Check sheet for the modelled part. Datum: model origin and axes. Units: mm. Round coordinates to 2 decimals unless told otherwise and drop trailing zeros. Order: outer loops, then holes, each group sorted by start corner. A loop starts at its lowest first (then second) coordinate and runs counter-clockwise, first axis right, second up.
Q1. Cross-section at B-B on y = 2. Give the number of separate pieces and of enclosed holes in the cut face, then the cut area to 3 significant figures.
Q2. Scan lines: probe 1 along Z at (x, y) = (5, 3.5); probe 2 along Y at (x, z) = (10.5, 1.95); probe 3 along Y at (x, z) = (7.25, 2.05). Record each from-to range of solid material in increasing order.
Q3. Cross-section at A-A on x = 12.25. Record the cut outline in (y, z).
Q4. Depth check by flat-ended pin: P1, Ø1.2, axis at x = 2.5, z = 1, coming from the +Y side. Enter the tip coordinate at first touch or a pass-through.
Q5. Mould release check, pull along Z, two halves, no side actions. Record for faces 1 (the flat face through (7, 0, 0.5)), 2 (the flat face through (9, 0, 2.5)): +Z half, -Z half, draft (parallel to the pull), parting line (faces both ways), or undercut.
from build123d import *

# Parameters (mm, degrees)
SKETCH1_W                  = 2.5
SKETCH1_H                  = 8
BOSS_EXTRUDE1_DEPTH        = 2.5
SKETCH2_W                  = 1.5
SKETCH2_H                  = 1.5
CUT_EXTRUDE2_DEPTH         = 7
CHAMFER3_SIZE              = 0.25
LPATTERN2_COUNT            = 8
LPATTERN2_PITCH            = 2.5
CHAMFER3_OF_LPATTERN2_SIZE = 0.25


with BuildPart() as part:
    # Sketch1 → Boss-Extrude1 (new body)
    with BuildSketch(Plane.XY):
        Rectangle(SKETCH1_W, SKETCH1_H)
    boss_extrude1 = extrude(amount=BOSS_EXTRUDE1_DEPTH)

    # Sketch2 → Cut-Extrude2 (cut)
    with BuildSketch(Plane(origin=(0, 4, 0), x_dir=(1, 0, 0), z_dir=(0, 1, 0))):
        with Locations((0, -1.25)):
            Rectangle(SKETCH2_W, SKETCH2_H)
    cut_extrude2 = extrude(amount=-CUT_EXTRUDE2_DEPTH, mode=Mode.SUBTRACT)

    # Chamfer3
    chamfer3_edges = [part.edges().sort_by_distance(p)[0] for p in [
        (0, 4, 2),
        (0.75, 4, 1.25),
        (0, 4, 0.5),
        (-0.75, 4, 1.25),
    ]]
    chamfer(chamfer3_edges, length=CHAMFER3_SIZE)

    # LPattern2: Boss-Extrude1, Cut-Extrude2 ×8
    with Locations(*[(i * LPATTERN2_PITCH, 0, 0) for i in range(1, LPATTERN2_COUNT)]):
        add(boss_extrude1)
        add(cut_extrude2, mode=Mode.SUBTRACT)

    # Chamfer3 of LPattern2
    chamfer3_of_lpattern2_edges = [part.edges().sort_by_distance(p)[0] for p in [
        (2.5, 4, 2),
        (3.25, 4, 1.25),
        (2.5, 4, 0.5),
        (1.75, 4, 1.25),
        (5, 4, 2),
        (5.75, 4, 1.25),
        (5, 4, 0.5),
        (4.25, 4, 1.25),
        (7.5, 4, 2),
        (8.25, 4, 1.25),
        (7.5, 4, 0.5),
        (6.75, 4, 1.25),
        (10, 4, 2),
        (10.75, 4, 1.25),
        (10, 4, 0.5),
        (9.25, 4, 1.25),
        (12.5, 4, 2),
        (13.25, 4, 1.25),
        (12.5, 4, 0.5),
        (11.75, 4, 1.25),
        (15, 4, 2),
        (15.75, 4, 1.25),
        (15, 4, 0.5),
        (14.25, 4, 1.25),
        (17.5, 4, 2),
        (18.25, 4, 1.25),
        (17.5, 4, 0.5),
        (16.75, 4, 1.25),
    ]]
    chamfer(chamfer3_of_lpattern2_edges, length=CHAMFER3_OF_LPATTERN2_SIZE)


solid = part.part
Results found:
1. separate pieces: 1
1. enclosed holes: 8
1. area: 32.0 mm2
2. probe 1: z = 0 to 0.5, 2 to 2.5
2. probe 2: y = -4 to -3
2. probe 3: y = -4 to 3.8
3. outline: (-4, 0) - (4, 0) - (4, 0.25) - (3.75, 0.5) - (-3, 0.5) - (-3, 2) - (3.75, 2) - (4, 2.25) - (4, 2.5) - (-4, 2.5) - close
4. P1: stops at y = 3.85
5. face 1: undercut
5. face 2: +Z half
